Autodesk Inventor part; units mm, degrees
ref_plane "YZ Plane" through (0, 0, 0) normal (1, 0, 0) x (0, 1, 0)
ref_plane "XZ Plane" through (0, 0, 0) normal (0, 1, 0) x (-1, 0, 0)
ref_plane "XY Plane" through (0, 0, 0) normal (0, 0, 1) x (1, 0, 0)
sketch "Esboço1" plane through (0, 0, 0) normal (0, 1, 0) x (-1, 0, 0)
  line L0 (13, 26.5) -> (-13, 26.5) construction
  line L1 (-13, 26.5) -> (-13, -26.5) construction
  line L2 (-13, -26.5) -> (13, -26.5) construction
  line L3 (13, -26.5) -> (13, 26.5) construction
  line L4 (-18, 31.5) -> (18, 31.5)
  line L5 (18, 31.5) -> (18, -31.5)
  line L6 (18, -31.5) -> (-18, -31.5)
  line L7 (-18, -31.5) -> (-18, 31.5)
  line L8 (-18, 31.5) -> (18, -31.5) construction
  line L9 (18, 31.5) -> (-18, -31.5) construction
  circle A0 centre (9.25, 18.5) radius 1.45
  circle A1 centre (-9.5, -19) radius 1.45
  point P0 (0, 0)
  dimension "d0" = 53
  dimension "d1" = 26
  dimension "d2" = 26.5
  dimension "d3" = 13
  dimension "d4" = 5
  dimension "d5" = 5
  dimension "d6" = 2.9
  dimension "d7" = 2.9
  dimension "d10" = 45
  dimension "d11" = 3.75
  dimension "d12" = 45.5
  dimension "d13" = 3.5
extrude "Extrusão1" add sketch "Esboço1" along normal blind 10 contours L4 L5 L6 L7 | A0 | A1
sketch "Esboço2" plane through (0, 10, 0) normal (0, 1, 0) x (1, 0, 0)
  circle A0 centre (-9.25, -18.5) radius 1.45
  circle A1 centre (9.5, 19) radius 1.45
  point P0 (0, 0)
extrude "Extrusão2" cut sketch "Esboço2" against normal blind 8.5
fillet "Arredondamento1" radius 5 4 edges at (18, 5, 31.5) (18, 5, -31.5) (-18, 5, -31.5) (-18, 5, 31.5)
equation "\"d7\" = d6"
properties part number "BASE BUCKBOOST"
Work out the finished part from the listing and answer in its coordinate system (mm). A direction names the side the tool comes from. Round coordinates to 2 decimals unless told otherwise and drop trailing zeros. Loops run counter-clockwise (first coordinate to the right, second up) from the corner with the lowest first, then second, coordinate; pieces in that order, holes last. Notation, with made-up numbers: (-21, -40) -> (17, -40) arc R21 ccw to (17, -6) -> close; hole circle Ø8 at (69.5, 0). An arc over 180 degrees is marked (long way). Write each question's results on one line, items separated by ' | '. Start each with the question number.
1. Section A-A (y = 4.25) is taken. Determine the outline of the cut face in (x, z), plus the area to 3 significant figures.
2. Given pin 1 Ø1.7 at (x, z) = (-9.25, 18.5) entering from +Y, flat-ended and moving along its own axis, determine where the tip first touches the part or whether it passes through.
3. Section B-B (x = -9.25) is taken. Determine the outline of the cut face in (y, z).
4. Find the intervals of material crossed by probe 1 along Z at (x, y) = (-9.25, 3.75); probe 2 along Z at (x, y) = (9.5, 6); probe 3 along X at (y, z) = (7.5, -19), in increasing order. Write a range as from..to.
5. For a pull along X with two mould halves and no side action, classify faces 3 (the face through (0, 5, 31.5)), 4 (the face through (16.57, 5.07, -30)), 5 (the face through (9, 1.5, -19)), 6 (the face through (-18, 5, 0)) as +X half, -X half, draft (parallel to the pull), parting line (faces both ways), or undercut.
6. A tool of negligible diameter and unlimited length cuts with its end or side. For faces 1 (the face through (0, 5, -31.5)), 2 (the face through (-9, 1.5, 18)), from which of +Z, -Z, +X, -X, +Y, -Y can it reach the whole face along a straight path? Write none if from no direction.
Evaluation:
1) outline: (-18, -26.5) arc R5 ccw to (-13, -31.5) -> (13, -31.5) arc R5 ccw to (18, -26.5) -> (18, 26.5) arc R5 ccw to (13, 31.5) -> (-13, 31.5) arc R5 ccw to (-18, 26.5) -> close; hole circle Ø2.9 at (-9.25, 18.5); hole circle Ø2.9 at (9.5, -19) | area: 2,230 mm2
2) pin 1: stops at y = 1.5
3) outline: (0, -31.5) -> (10, -31.5) -> (10, 17.05) -> (1.5, 17.05) -> (1.5, 19.95) -> (10, 19.95) -> (10, 31.5) -> (0, 31.5) -> close
4) probe 1: z = -31.5..17.05, 19.95..31.5 | probe 2: z = -31.5..-20.45, -17.55..31.5 | probe 3: x = -18..8.05, 10.95..18
5) face 3: draft | face 4: +X half | face 5: undercut | face 6: -X half
6) face 1: -Z, +X, -X, +Y, -Y | face 2: +Y
